Verification items for the finished model (mm, model axes). A direction names the side the tool comes from. Round coordinates to 2 decimals unless told otherwise and drop trailing zeros. Write each loop counter-clockwise with the first axis right and the second up, starting at its lowest first coordinate (ties: lowest second). Pieces come first, ordered by that corner, then holes. Notation, with made-up numbers: M -4,60 L 18,60 A8 ccw 18,74 Z; hole C -34.5,49.5 d10. An arc over 180 degrees is marked long. One line per item, written item: value. Start each with the question number.
from build123d import *

# Parameters (mm, degrees)
F0_W       = 146.05
F0_H       = 25.4
F1_DEPTH   = 38.1
F2_W       = 7.62
F2_H       = 12.7
F1_FACE1_W = 38.1
F1_FACE1_H = 25.4
F3_DEPTH   = 146.051
F5_DEPTH   = 25.401
F6_W       = 146.05
F6_H       = 15.24
F7_DEPTH   = 38.1
F8_W       = 9.0582419944
F8_H       = 15.24
F9_DEPTH   = 38.1
F10_W      = 2.4497217488
F10_H      = 15.24
F11_DEPTH  = 38.1
F12_R      = 3.96875
F13_DEPTH  = 38.101


with BuildPart() as f1:
    # F0 (on Front) → F1 (new body)
    with BuildSketch(Plane.XZ):
        with Locations((-17.8064775685, -20.8892399079)):
            Rectangle(F0_W, F0_H)
    extrude(amount=F1_DEPTH)

    # F2 (on face) + F1_face1 (on face) → F3 (cut, through all)
    with BuildSketch(Plane(origin=(-90.8314775685, 0, 0), x_dir=(0, -1, 0), z_dir=(-1, 0, 0))):
        with Locations((19.05, -14.5392399079)):
            Rectangle(F2_W, F2_H)
    with BuildSketch(Plane(origin=(55.2185224315, -19.05, -20.8892399079), x_dir=(0, 1, 0), z_dir=(1, 0, 0))):
        Rectangle(F1_FACE1_W, F1_FACE1_H)
    extrude(amount=-F3_DEPTH, dir=(-1, 0, 0), mode=Mode.SUBTRACT)

    # F4 (on face) → F5 (cut, through all)
    with BuildSketch(Plane.XY.offset(-8.1892399079)):
        Polygon((52.7688006827, -22.86), (-81.7732355741, -22.86), (-81.7732355741, -38.1), (52.7688006827, -38.1), (52.7688006827, -30.48), align=None)
    extrude(amount=-F5_DEPTH, mode=Mode.SUBTRACT)

    # F6 (on face) → F7 (join)
    with BuildSketch(Plane.XY.offset(-8.1892399079)):
        with Locations((-17.8064775685, -7.62)):
            Rectangle(F6_W, F6_H)
    extrude(amount=F7_DEPTH)

    # F8 (on face) → F9 (join)
    with BuildSketch(Plane.XY.offset(-8.1892399079)):
        with Locations((-86.3023565713, -30.48)):
            Rectangle(F8_W, F8_H)
    extrude(amount=F9_DEPTH)

    # F10 (on face) → F11 (join)
    with BuildSketch(Plane.XY.offset(-8.1892399079)):
        with Locations((53.9936615571, -30.48)):
            Rectangle(F10_W, F10_H)
    extrude(amount=F11_DEPTH)

    # F12 (on face) → F13 (cut, through all)
    with BuildSketch(Plane(origin=(0, 0, 0), x_dir=(-1, 0, 0), z_dir=(0, 1, 0))):
        with Locations((-44.652171433, -33.5892399079)):
            Circle(F12_R)
        with BuildLine():
            ThreePointArc((66.466478567, -33.5892399079), (70.441578567, -37.5643399079), (74.416678567, -33.5892399079))
            ThreePointArc((74.416678567, -33.5892399079), (70.441578567, -29.6141399079), (66.466478567, -33.5892399079))
        make_face()
    extrude(amount=-F13_DEPTH, mode=Mode.SUBTRACT)


solid = f1.part
1) Cross-section at A-A (z = 20). Record the boundary of the cut face in (x, y).
2) Mould release check, pull along X, two halves, no side actions. Record for faces 4 (the flat face through (-81.773, -31, -2)), 5 (the flat face through (55.219, -24, -2)), 6 (the flat face through (53, -15, -33.589)), 7 (the flat face through (52.769, -31, -2)): pulls with the +X half, pulls with the -X half, needs draft (parallel to the pull), parting line crosses it, or undercut.
3) Cross-section at D-D (y = -18). Record the boundary of the cut face in (x, z), then the cut area to 3 significant figures.
4) Cross-section at B-B (y = -29). Record the boundary of the cut face in (x, z).
5) Gauge pin test, flat ends, axial feed: pin 1 Ø14 at (x, z) = (-25, -25.5) entering from -Y; pin 2 Ø4 at (x, y) = (-40, -20.5) entering from +Z; pin 3 Ø15 at (x, z) = (-48, 13) entering from -Y. Record the tip position at first contact, or that the pin passes through.
6) Thickness scan on line 1 (X direction, y = -31.5, z = -7.5); line 2 (Y direction, x = -6, z = -7); line 3 (Z direction, x = -62, y = -21). Record the ranges inside material, lowest first.
7) Access from +Z, -Z, +X, -X, +Y, -Y to the whole of each face (thin tool, end or side, straight path). Record for faces 1 (the flat face through (-86, -22.86, 4)), 2 (the flat face through (-14, -22.86, -27)), 3 (the flat face through (-14, -11, -33.589)).
8) Cross-section at C-C (x = -34.5). Record the boundary of the cut face in (y, z).
Results below:
1. outline: M -90.83,-38.1 L -81.77,-38.1 L -81.77,-22.86 L -90.83,-22.86 Z; M -90.83,-15.24 L 55.22,-15.24 L 55.22,0 L -90.83,0 Z; M 52.77,-38.1 L 55.22,-38.1 L 55.22,-22.86 L 52.77,-22.86 Z
2. face 4: undercut
2. face 5: pulls with the +X half
2. face 6: needs draft
2. face 7: undercut
3. outline: M -90.83,-33.59 L -74.42,-33.59 A3.98 cw -66.47,-33.59 L 40.68,-33.59 A3.97 cw 48.62,-33.59 L 55.22,-33.59 L 55.22,-20.89 L -90.83,-20.89 Z
3. area: 1,810 mm²
4. outline: M -90.83,-33.59 L -81.77,-33.59 L -81.77,29.91 L -90.83,29.91 Z; M 52.77,-33.59 L 55.22,-33.59 L 55.22,29.91 L 52.77,29.91 Z
5. pin 1: stops at y = -22.86
5. pin 2: stops at z = -20.89
5. pin 3: stops at y = -15.24
6. line 1: x = -90.83 to -81.77, 52.77 to 55.22
6. line 2: y = -15.24 to 0
6. line 3: z = -33.59 to -20.89
7. face 1: +Z, +X, -X
7. face 2: +Z, -Z, -Y
7. face 3: -Z, +X, -X, +Y, -Y
8. outline: M -22.86,-33.59 L 0,-33.59 L 0,29.91 L -15.24,29.91 L -15.24,-20.89 L -22.86,-20.89 Z
